Design review of the part built by this model. Coordinates are the model's own, in mm. Round coordinates to 2 decimals unless told otherwise and drop trailing zeros. Order: outer loops, then holes, each group sorted by start corner. A loop starts at its lowest first (then second) coordinate and runs counter-clockwise, first axis right, second up.
Autodesk Inventor part; units mm, degrees
ref_plane "YZ Plane" through (0, 0, 0) normal (1, 0, 0) x (0, 1, 0)
ref_plane "XZ Plane" through (0, 0, 0) normal (0, 1, 0) x (-1, 0, 0)
ref_plane "XY Plane" through (0, 0, 0) normal (0, 0, 1) x (1, 0, 0)
sketch "草圖1" plane through (0, 0, 0) normal (0, 0, 1) x (1, 0, 0)
  line L0 (0, -20.605) -> (0, 20.605) construction
  line L1 (2, -20.605) -> (2, 20.605)
  line L2 (-2, 20.605) -> (-2, -20.605)
  arc A0 (-2, -20.605) -> (2, -20.605) centre (0, -20.605) ccw
  arc A1 (2, 20.605) -> (-2, 20.605) centre (0, 20.605) ccw
  point P0 (0, 0)
  dimension "d0" = 41.21
  dimension "d1" = 4
extrude "擠出1" add sketch "草圖1" along normal blind 1
sketch "草圖2" plane through (0, 0, 1) normal (0, 0, 1) x (1, 0, 0)
  arc A0 (-2, -20.605) -> (2, -20.605) centre (0, -20.605) ccw
  circle A1 centre (0, -20.605) radius 0.75
  arc A2 (2, 20.605) -> (-2, 20.605) centre (0, 20.605) ccw
  circle A3 centre (0, 20.605) radius 0.75
  point P0 (0, 0)
  dimension "d4" = 1.5
  dimension "d5" = 1.5
extrude "擠出2" add sketch "草圖2" along normal blind 1
sketch "草圖3" plane through (0, 0, 1) normal (0, 0, 1) x (1, 0, 0)
  circle A0 centre (0, 20.605) radius 0.75
  circle A1 centre (0, -20.605) radius 0.75
  circle A2 centre (0, 20.605) radius 1
  circle A3 centre (0, -20.605) radius 0.75
  circle A4 centre (0, -20.605) radius 1
  point P0 (0, 0)
  dimension "d8" = 2
  dimension "d9" = 2
extrude "擠出3" cut sketch "草圖3" along normal mid plane 10 contours A0 | A1 | A2 | A4
sketch "草圖4" plane through (0, 0, 1) normal (0, 0, 1) x (1, 0, 0)
  line L0 (-2, 20.605) -> (-2, -20.605)
  arc A0 (-2, -15.8965) -> (-2, -5.3135) centre (-8, -10.605) ccw
  circle A1 centre (0, -20.605) radius 1
  point P0 (0, 0)
  dimension "d12" = 8
  dimension "d13" = 6
  dimension "d14" = 10
extrude "擠出4" cut sketch "草圖4" along normal mid plane 10 contours A0 L0
properties part number "連桿3"
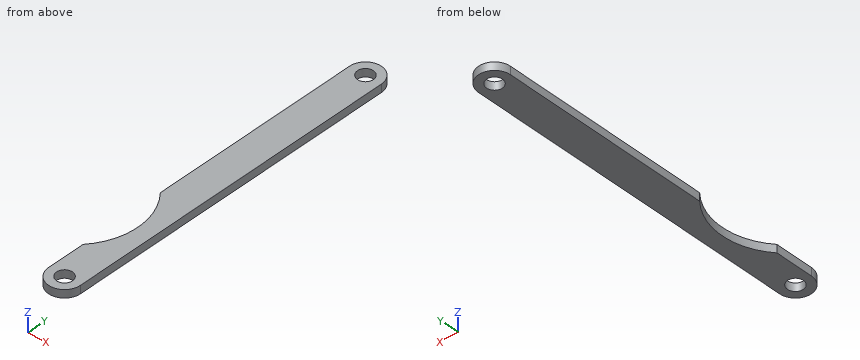
1) Take a section at B-B on x = 1.6. Give the boundary of the cut face in (y, z) (3 decimals).
Results:
outline: (-21.805, 0) - (21.805, 0) - (21.805, 1) - (-21.805, 1) - close
2) Take a section at A-A on z = 0.85. Give the boundary of the cut face in (x, y) (1 decimal), plus the area to 3 significant figures.
Results:
outline: (-2, -20.6) arc R2 ccw to (2, -20.6) - (2, 20.6) arc R2 ccw to (-2, 20.6) - (-2, -5.3) arc R8 cw to (-2, -15.9) - close; hole circle Ø2 at (0, -20.6); hole circle Ø2 at (0, 20.6)
area: 157 mm2
3) Clearance check with a flat-ended pin moving along its axis: P1, Ø2, axis at x = -1.5, y = -9, coming from the -Z side. State where the tip first meets the part, or that it passes through.
Results:
P1: passes through
4) To check wall thickness, follow line 1 along Y through (x, z) = (0.2, 0.45); line 2 along Y through (x, z) = (-0.6, 0.95) (3 decimals); line 3 along Y through (x, z) = (-1.75, 0.25). State the ranges of each line that lie inside material, in increasing order.
Results:
line 1: y = -22.59 to -21.58, -19.63 to 19.63, 21.58 to 22.59
line 2: y = -22.513 to -21.405, -19.805 to -13.645, -7.565 to 19.805, 21.405 to 22.513
line 3: y = -21.57 to -15.6, -5.61 to 21.57
